Input: part model. Units: mm. Frame: model coordinates. Face numbers are marked on the shaded views. A direction names the side the tool comes from. Coordinates: 2 decimals unless noted, no trailing zeros. Loops run counter-clockwise (first coordinate to the right, second up) from the corner with the lowest first, then second, coordinate; pieces in that order, holes last.
```python
from build123d import *

# Parameters (mm, degrees)
SKETCH2_R           = 11.475
BOSS_EXTRUDE1_DEPTH = 11.225
SKETCH5_R           = 10.98
BOSS_EXTRUDE3_DEPTH = 1.7
SKETCH6_R           = 1.5
CUT_EXTRUDE4_DEPTH  = 5


with BuildPart() as part:
    # Sketch1 → Revolve1 (revolve)
    with BuildSketch(Plane(origin=(0, 0, 0), x_dir=(1, 0, 0), z_dir=(0, 1, 0))):
        with BuildLine():
            Line((0, 9.525), (0, -9.525))
            ThreePointArc((0, -9.525), (9.525, 0), (0, 9.525))
        make_face()
    revolve(axis=Axis((0, 0, -9.525), (0, 0, 1)))

    # Sketch2 → Boss-Extrude1 (add)
    with BuildSketch(Plane(origin=(0, 0, 0), x_dir=(1, 0, 0), z_dir=(0, 1, 0))):
        with Locations(Location((0, 0, 0), (0, 0, 270))):
            Circle(SKETCH2_R)
    extrude(amount=BOSS_EXTRUDE1_DEPTH)

    # Sketch5 → Boss-Extrude3 (add)
    with BuildSketch(Plane(origin=(0, 11.225, 0), x_dir=(1, 0, 0), z_dir=(0, 1, 0))):
        with Locations(Location((0, 0, 0), (0, 0, 270))):
            Circle(SKETCH5_R)
    extrude(amount=BOSS_EXTRUDE3_DEPTH)

    # Sketch6 → Cut-Extrude4 (cut)
    with BuildSketch(Plane(origin=(0, 12.925, 0), x_dir=(1, 0, 0), z_dir=(0, 1, 0))):
        with Locations(Location((7.747, 0, 0), (0, 0, 270))):
            Circle(SKETCH6_R)
        with Locations(Location((-7.747, 0, 0), (0, 0, 270))):
            Circle(SKETCH6_R)
    extrude(amount=-CUT_EXTRUDE4_DEPTH, mode=Mode.SUBTRACT)


solid = part.part
```
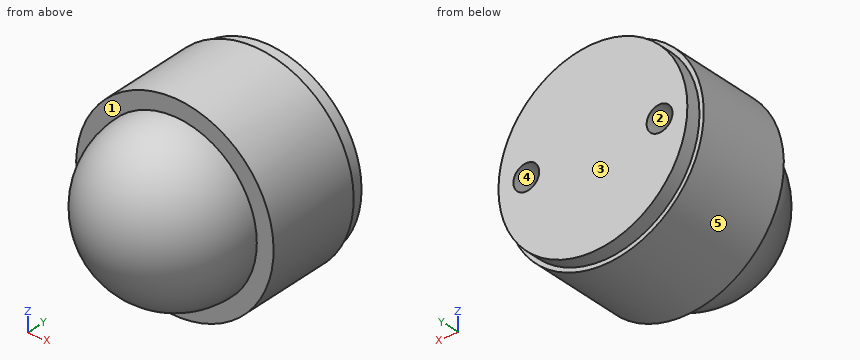
Item 1: Section query A-A (x = 0). Output: boundary loops of the cut face in (y, z) (3 decimals).
Result:
outline: (0, -11.475) - (11.225, -11.475) - (11.225, -10.98) - (12.925, -10.98) - (12.925, 10.98) - (11.225, 10.98) - (11.225, 11.475) - (0, 11.475) - (0, 9.525) arc R9.525 ccw to (0, -9.525) - close
Item 2: Section query B-B (z = 0). Output: boundary loops of the cut face in (x, y) (3 decimals), then the cut area to 3 significant figures.
Result:
outline: (-11.475, 0) - (-9.525, 0) arc R9.525 ccw to (9.525, 0) - (11.475, 0) - (11.475, 11.225) - (10.98, 11.225) - (10.98, 12.925) - (9.247, 12.925) - (9.247, 7.925) - (6.247, 7.925) - (6.247, 12.925) - (-6.247, 12.925) - (-6.247, 7.925) - (-9.247, 7.925) - (-9.247, 12.925) - (-10.98, 12.925) - (-10.98, 11.225) - (-11.475, 11.225) - close
area: 407 mm2
Item 3: Contact query for flat-ended pins moving along their axis: P1, Ø4, axis at x = -4.5, y = 5.5, coming from the +Z side; P2, Ø11.5, axis at x = -4.5, z = 0.5, coming from the -Y side (3 decimals); P3, Ø3, axis at y = -3, z = -7, coming from the +X side; P4, Ø2.5, axis at x = -7.5, z = 0.5, coming from the +Y side (3 decimals). Output: stop coordinate, or through.
Result:
P1: stops at z = 11.2
P2: stops at y = -9.525
P3: stops at x = 7.3
P4: stops at y = 12.925
Item 4: Section query C-C (y = 2.5). Output: boundary loops of the cut face in (x, z) (3 decimals), then the cut area to 3 significant figures.
Result:
outline: circle Ø22.95 at (0, 0)
area: 414 mm2
Item 5: Mould query, pull axis Z, two halves, no side actions, for the marked faces 3, 4 and 5. Classes: +Z half, -Z half, draft (parallel to the pull), parting line (faces both ways), or undercut.
Result:
face 3: draft
face 4: undercut
face 5: parting line
Item 6: Section query D-D (x = 3). Output: boundary loops of the cut face in (y, z) (3 decimals), then the cut area to 3 significant figures.
Result:
outline: (0, -11.076) - (11.225, -11.076) - (11.225, -10.562) - (12.925, -10.562) - (12.925, 10.562) - (11.225, 10.562) - (11.225, 11.076) - (0, 11.076) - (0, 9.04) arc R9.04 ccw to (0, -9.04) - close
area: 413 mm2
Item 7: Reachability of the marked faces 1 and 2 from +Z, -Z, +X, -X, +Y, -Y: full face, straight path, thin tool, end or side. Return the list, or none.
Result:
face 1: -Y
face 2: +Y
Item 8: Line query: L1, parallel to X at y = 10, z = 0 (3 decimals); L2, parallel to X at y = 11.55, z = 0; L3, parallel to Y at x = -9.25, z = -3.5 (3 decimals). Output: solid intervals per line, ascending.
Result:
L1: x = -11.475 to -9.247, -6.247 to 6.247, 9.247 to 11.475
L2: x = -10.98 to -9.25, -6.25 to 6.25, 9.25 to 10.98
L3: y = 0 to 12.925
